```python
from build123d import *

# Parameters (mm, degrees)
BOSS_EXTRU_2_DEPTH           = 5
ESQUISSE2_R                  = 1.5
ENL_V_MAT_EXTRU_1_DEPTH      = 5
R_P_TITION_CIRCULAIRE1_COUNT = 6
ESQUISSE3_R                  = 6.25
ENL_V_MAT_EXTRU_2_DEPTH      = 5
ESQUISSE4_W                  = 5
ESQUISSE4_H                  = 5
ENL_V_MAT_EXTRU_3_DEPTH      = 10
R_P_TITION_LIN_AIRE1_COUNT   = 4
R_P_TITION_LIN_AIRE1_PITCH   = 10
ESQUISSE5_W                  = 11.156910716
ESQUISSE5_H                  = 32.673754016
ESQUISSE5_W_2                = 16.593305943
ENL_V_MAT_EXTRU_4_DEPTH      = 10


with BuildPart() as part:
    # Esquisse1 → Boss.-Extru.2 (new body)
    with BuildSketch(Plane.XY):
        with BuildLine():
            ThreePointArc((18.5, 0), (0, -18.5), (-18.5, 0))
            Line((-18.5, 0), (-25, 28.75))
            Line((-25, 28.75), (25, 28.75))
            Line((25, 28.75), (18.5, 0))
        make_face()
    extrude(amount=BOSS_EXTRU_2_DEPTH)

    # Esquisse2 → Enlèv. mat.-Extru.1 (cut)
    with BuildSketch(Plane.XY.offset(5)):
        with Locations((-7.75, -13.423393759)):
            Circle(ESQUISSE2_R)
    enl_v_mat_extru_1 = extrude(amount=-ENL_V_MAT_EXTRU_1_DEPTH, mode=Mode.SUBTRACT)

    # Répétition circulaire1: Enlèv. mat.-Extru.1 ×6 about axis
    r_p_tition_circulaire1_axis = Axis((0, 0, 0), (0, 0, 1))
    for i in range(1, R_P_TITION_CIRCULAIRE1_COUNT):
        add(enl_v_mat_extru_1.rotate(r_p_tition_circulaire1_axis, i * 360 / R_P_TITION_CIRCULAIRE1_COUNT), mode=Mode.SUBTRACT)

    # Esquisse3 → Enlèv. mat.-Extru.2 (cut)
    with BuildSketch(Plane.XY.offset(5)):
        with Locations((0, 7)):
            Circle(ESQUISSE3_R)
    extrude(amount=-ENL_V_MAT_EXTRU_2_DEPTH, mode=Mode.SUBTRACT)

    # Esquisse4 → Enlèv. mat.-Extru.3 (cut)
    with BuildSketch(Plane.XY.offset(5)):
        with Locations((-15, 26.25)):
            Rectangle(ESQUISSE4_W, ESQUISSE4_H)
    enl_v_mat_extru_3 = extrude(amount=-ENL_V_MAT_EXTRU_3_DEPTH, mode=Mode.SUBTRACT)

    # Répétition linéaire1: Enlèv. mat.-Extru.3 ×4
    with Locations(*[(i * R_P_TITION_LIN_AIRE1_PITCH, 0, 0) for i in range(1, R_P_TITION_LIN_AIRE1_COUNT)]):
        add(enl_v_mat_extru_3, mode=Mode.SUBTRACT)

    # Esquisse5 → Enlèv. mat.-Extru.4 (cut)
    with BuildSketch(Plane.XY.offset(5)):
        with Locations((28.078455358, 23.582495232)):
            Rectangle(ESQUISSE5_W, ESQUISSE5_H)
        with Locations((-30.796652972, 23.582495232)):
            Rectangle(ESQUISSE5_W_2, ESQUISSE5_H)
    extrude(amount=-ENL_V_MAT_EXTRU_4_DEPTH, mode=Mode.SUBTRACT)


solid = part.part
```
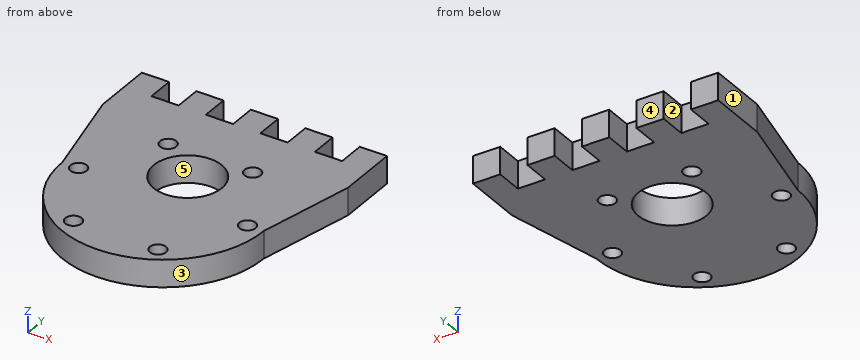
Here's how the part is built. I have some questions about the finished solid (model axes, mm). Face numbers are marked on the shaded views. A direction names the side the tool comes from. Give positions to 0.01 mm unless a question says otherwise; leave off trailing zeros. Order: outer loops, then holes, each group sorted by start corner. A loop starts at its lowest first (then second) coordinate and runs counter-clockwise, first axis right, second up. Notation, with made-up numbers: (-35, -5.5) - (-7, -5.5) arc R17 ccw to (-7, 10.5) - close; hole circle Ø5 at (-13.75, -12.75). An arc over 180 degrees is marked (long way). Answer as a JSON object with one key per item and string values. Group by question number.
Item 1: Which directions (+Z, -Z, +X, -X, +Y, -Y) give clear straight access to the entire face, cutting with the end or side of a thin tool? Please do the marked faces 1 and 2.
Item 2: Please list where these lines run through material, in increasing order: probe 1 along X at (y, z) = (-0.5, 3.5); probe 2 along Y at (x, z) = (-16, 2.85); probe 3 along Y at (x, z) = (7.75, 2.5).
Item 3: For P1, Ø1.8, axis at x = 7.75, y = 13.42, coming from the -Z side; P2, Ø2, axis at y = 13, z = 3, coming from the -X side; P3, Ø1.5, axis at x = -5.5, z = 1.5, coming from the +Y side, each with a flat end and sliding along its axis, tell me the tip position at first contact or that it passes through.
Item 4: If we section it at C-C on z = 2.65: Give the number of separate pieces and of enclosed holes in the cut face, and give its area (3 significant figures).
Item 5: If we section it at D-D on x = -11.5: Please give me the cut outline in (y, z), and give its area (3 significant figures).
Item 6: If we section it at B-B on y = 8: Please give me the cut outline in (x, z), and give its area (3 significant figures).
Item 7: If we section it at A-A on x = 0: Please give me the cut outline in (y, z).
Item 8: If we mould it in two halves opening along X, with no side actions, what happens to the marked faces 3, 4 and 5? For each: pulls with the +X half, pulls with the -X half, needs draft (parallel to the pull), parting line crosses it, or undercut.
Result set:
{
 "1": {"face 1": "+Z, -Z, -X, +Y, -Y", "face 2": "+Z, -Z, +Y"},
 "2": {"probe 1": "-18.49 to -16.91, -14.09 to 14.09, 16.91 to 18.49", "probe 2": "-9.29 to -1.41, 1.41 to 23.75", "probe 3": "-16.8 to -14.92, -11.92 to 11.92, 14.92 to 28.75"},
 "3": {"P1": "through", "P2": "x = -21.67", "P3": "y = 23.75"},
 "4": {"separate pieces": "1", "enclosed holes": "7", "area": "1,500 mm²"},
 "5": {"outline": "(-14.49, 0) - (28.75, 0) - (28.75, 5) - (-14.49, 5) - close", "area": "216 mm²"},
 "6": {"outline": "(-20.31, 0) - (-6.17, 0) - (-6.17, 5) - (-20.31, 5) - close; (6.17, 0) - (20.31, 0) - (20.31, 5) - (6.17, 5) - close", "area": "141 mm²"},
 "7": {"outline": "(-18.5, 0) - (0.75, 0) - (0.75, 5) - (-18.5, 5) - close; (13.25, 0) - (28.75, 0) - (28.75, 5) - (13.25, 5) - close"},
 "8": {"face 3": "parting line crosses it", "face 4": "needs draft", "face 5": "undercut"}
}
